Build history of the part. All positions in model axes, mm. A direction names the side the tool comes from. Round coordinates to 2 decimals unless told otherwise and drop trailing zeros. Order: outer loops, then holes, each group sorted by start corner. A loop starts at its lowest first (then second) coordinate and runs counter-clockwise, first axis right, second up. Notation, with made-up numbers: M 39.25,43.25 L 47.25,43.25 A21 cw 47.25,80.25 Z; hole C 40.25,-26.5 d11. An arc over 180 degrees is marked long. Use CSV: the item, a comma, the result in double quotes.
from build123d import *

# Parameters (mm, degrees)
F0_W     = 110.066666
F0_H     = 31.8
F0_R     = 2.125
F1_DEPTH = 6.4
F2_W     = 110.066666
F2_H     = 38.2
F2_R     = 2.125
F3_DEPTH = 6.4
F4_SIZE  = 1.5


with BuildPart() as f1:
    # F0 (on Top) → F1 (new body)
    with BuildSketch(Plane.XY):
        Rectangle(F0_W, F0_H)
        with Locations((-39.033333, 6.5)):
            Circle(F0_R, mode=Mode.SUBTRACT)
        with Locations((0, 6.5)):
            Circle(F0_R, mode=Mode.SUBTRACT)
        with Locations((39.033333, 6.5)):
            Circle(F0_R, mode=Mode.SUBTRACT)
    extrude(amount=F1_DEPTH)

    # F2 (on face) → F3 (join)
    with BuildSketch(Plane.XZ.offset(15.9)):
        with Locations((0, 19.1)):
            Rectangle(F2_W, F2_H)
        with Locations((-39.033333, 22.4)):
            Circle(F2_R, mode=Mode.SUBTRACT)
        with Locations((0, 22.4)):
            Circle(F2_R, mode=Mode.SUBTRACT)
        with Locations((39.033333, 22.4)):
            Circle(F2_R, mode=Mode.SUBTRACT)
    extrude(amount=F3_DEPTH)

    # F4
    f4_edges = [f1.edges().sort_by_distance(p)[0] for p in [
        (0, -22.3, 38.2),
        (0, -22.3, 0),
        (0, 15.9, 0),
        (55.033333, -3.2, 0),
        (55.033333, 15.9, 3.2),
        (-55.033333, 15.9, 3.2),
        (-55.033333, -3.2, 0),
        (-55.033333, -22.3, 19.1),
        (55.033333, -22.3, 19.1),
        (-55.033333, -19.1, 38.2),
        (55.033333, -19.1, 38.2),
    ]]
    chamfer(f4_edges, length=F4_SIZE)


solid = f1.part
(1) Wall check: line 1 (X direction, y = -18, z = 22); line 2 (Z direction, x = 0, y = -18) (3 decimals); line 3 (X direction, y = 6, z = 4). Give the ranges that are in metal, low to high. Write a range as from..to.
Answer block:
line 1,"x = -55.03..-41.12, -36.95..-2.09, 2.09..36.95, 41.12..55.03"
line 2,"z = 0..20.275, 24.525..38.2"
line 3,"x = -55.03..-41.1, -36.97..-2.07, 2.07..36.97, 41.1..55.03"
(2) Cut at A-A, the plane z = 22.4. Give the cut face in (x, y) (3 decimals), and give its area (3 significant figures).
Answer block:
outline,"M -55.033,-20.8 L -53.533,-22.3 L -41.158,-22.3 L -41.158,-15.9 L -55.033,-15.9 Z; M -36.908,-22.3 L -2.125,-22.3 L -2.125,-15.9 L -36.908,-15.9 Z; M 2.125,-22.3 L 36.908,-22.3 L 36.908,-15.9 L 2.125,-15.9 Z; M 41.158,-22.3 L 53.533,-22.3 L 55.033,-20.8 L 55.033,-15.9 L 41.158,-15.9 Z"
area,"621 mm²"
(3) Two-plate mould, pull along X, no slides. Class faces 1 (the face through (55.033, -10, 6)), 2 (the face through (-1, 0, 6.4)), 3 (the face through (40.18, -19.06, 24.19)): released by +X, released by -X, zero draft, split by the parting line, or undercut.
Answer block:
face 1,"released by +X"
face 2,"zero draft"
face 3,"undercut"
(4) Cut at D-D, the plane x = 46. Give the cut face in (y, z).
Answer block:
outline,"M -22.3,1.5 L -20.8,0 L 14.4,0 L 15.9,1.5 L 15.9,6.4 L -15.9,6.4 L -15.9,38.2 L -20.8,38.2 L -22.3,36.7 Z"
(5) Tool access for faces 4 (the face through (-1, 15.9, 4)), 5 (the face through (-1, -15.9, 26)): list every direction of +Z, -Z, +X, -X, +Y, -Y with a clear straight run to the whole face (end or side of a thin tool).
Answer block:
face 4,"+Z, -Z, +X, -X, +Y"
face 5,"+Z, +X, -X, +Y"
(6) Cut at B-B, the plane x = 0. Give the cut face in (y, z) (3 decimals), and give its area (3 significant figures).
Answer block:
outline,"M -22.3,1.5 L -20.8,0 L 4.375,0 L 4.375,6.4 L -15.9,6.4 L -15.9,20.275 L -22.3,20.275 Z; M -22.3,24.525 L -15.9,24.525 L -15.9,38.2 L -20.8,38.2 L -22.3,36.7 Z; M 8.625,0 L 14.4,0 L 15.9,1.5 L 15.9,6.4 L 8.625,6.4 Z"
area,"390 mm²"
(7) Cut at C-C, the plane y = 6.5. Give the cut face in (x, z) (3 decimals).
Answer block:
outline,"M -55.033,1.5 L -53.533,0 L -41.158,0 L -41.158,6.4 L -55.033,6.4 Z; M -36.908,0 L -2.125,0 L -2.125,6.4 L -36.908,6.4 Z; M 2.125,0 L 36.908,0 L 36.908,6.4 L 2.125,6.4 Z; M 41.158,0 L 53.533,0 L 55.033,1.5 L 55.033,6.4 L 41.158,6.4 Z"
(8) Drop flat-ended pins along their axis: pin 1 (3.5 mm diameter, centred on x = 0, y = 6.5, fed in from +Z); pin 2 (1 mm diameter, centred on x = -11.5, z = 8, fed in from +Y); pin 3 (4 mm diameter, centred on x = 8, y = -4, fed in from +Z); pin 4 (7 mm diameter, centred on x = 39.03, y = 6.5, fed in from -Z). Give the stop position or say it passes through.
Answer block:
pin 1,"passes through"
pin 2,"stops at y = -15.9"
pin 3,"stops at z = 6.4"
pin 4,"stops at z = 0"
